from build123d import *

# Parameters (mm, degrees)
SKETCH1_W               = 50
SKETCH1_H               = 91
SKETCH1_W_2             = 37.5
SKETCH1_W_3             = 25
BOSS_EXTRUDE1_DEPTH     = 25
SKETCH1_3_W             = 37.5
SKETCH1_3_H             = 91
BOSS_EXTRUDE2_DEPTH     = 35
BOSS_EXTRUDE3_REACH     = 66.013
SKETCH4_R               = 12.5
SKETCH4_R_2             = 6
SKETCH4_4_R             = 6
CUT_EXTRUDE1_DEPTH      = 65.01307477
SKETCH4_5_R             = 12.5
SKETCH4_5_R_2           = 6
BOSS_EXTRUDE4_DEPTH     = 15
SKETCH5_W               = 91
SKETCH5_H               = 60
BOSS_EXTRUDE5_DEPTH     = 15
CUT_EXTRUDE2_DEPTH      = 1
CUT_EXTRUDE2_DEPTH_BACK = 21
EXTRUDE_THIN1_DEPTH     = 21
BOSS_EXTRUDE6_REACH     = 88.811
SKETCH9_R               = 7.5
CUT_EXTRUDE4_DEPTH      = 5
SKETCH9_6_R             = 12.5
CUT_EXTRUDE5_DEPTH      = 5
SKETCH9_7_R             = 7.5
CUT_EXTRUDE6_DEPTH      = 87.810889132


with BuildPart() as part:
    # Sketch1 → Boss-Extrude1 (new body)
    with BuildSketch(Plane(origin=(0, 0, 0), x_dir=(0, 0, -1), z_dir=(0, 1, 0))):
        with Locations((25, 45.5)):
            Rectangle(SKETCH1_W, SKETCH1_H)
        with Locations((68.75, 45.5)):
            Rectangle(SKETCH1_W_2, SKETCH1_H)
        with Locations((100, 45.5)):
            Rectangle(SKETCH1_W_3, SKETCH1_H)
        with Locations((131.25, 45.5)):
            Rectangle(SKETCH1_W_2, SKETCH1_H)
        with Locations((175, 45.5)):
            Rectangle(SKETCH1_W, SKETCH1_H)
    extrude(amount=-BOSS_EXTRUDE1_DEPTH)

    # Sketch1<3> → Boss-Extrude2 (add)
    with BuildSketch(Plane(origin=(0, 0, 0), x_dir=(0, 0, -1), z_dir=(0, 1, 0))):
        with Locations((68.75, 45.5)):
            Rectangle(SKETCH1_3_W, SKETCH1_3_H)
        with Locations((131.25, 45.5)):
            Rectangle(SKETCH1_3_W, SKETCH1_3_H)
    extrude(amount=-BOSS_EXTRUDE2_DEPTH)

    # Boss-Extrude3: up to this face of the body (flat: up to its plane)
    boss_extrude3_end = Plane(part.part.faces().sort_by_distance((-45.5, 0, -100))[0])
    # Sketch4 → Boss-Extrude3 (add, up to the picked face)
    with BuildSketch(Plane(origin=(0, 0, 0), x_dir=(0.939692621, -0.342020143, 0), z_dir=(0.342020143, 0.939692621, 0)), mode=Mode.PRIVATE) as boss_extrude3_sk1:
        with BuildLine():
            ThreePointArc((-40, 15), (-65, 40), (-40, 65))
            Line((-40, 65), (0, 65))
            Line((0, 65), (0, 15))
            Line((0, 15), (-40, 15))
        make_face()
        with Locations((-40, 40)):
            Circle(SKETCH4_R, mode=Mode.SUBTRACT)
    boss_extrude3_tool1 = split(extrude(boss_extrude3_sk1.sketch, amount=-BOSS_EXTRUDE3_REACH, mode=Mode.PRIVATE), bisect_by=boss_extrude3_end, keep=Keep.BOTH, mode=Mode.PRIVATE)
    add(boss_extrude3_tool1.solids().sort_by_distance((-60.309415, 21.950832, -40))[0])
    # Sketch4 → Boss-Extrude3 (add, up to the picked face)
    with BuildSketch(Plane(origin=(0, 0, 0), x_dir=(0.939692621, -0.342020143, 0), z_dir=(0.342020143, 0.939692621, 0)), mode=Mode.PRIVATE) as boss_extrude3_sk2:
        with Locations((-40, 40)):
            Circle(SKETCH4_R)
        with Locations((-40, 40)):
            Circle(SKETCH4_R_2, mode=Mode.SUBTRACT)
    boss_extrude3_tool2 = split(extrude(boss_extrude3_sk2.sketch, amount=-BOSS_EXTRUDE3_REACH, mode=Mode.PRIVATE), bisect_by=boss_extrude3_end, keep=Keep.BOTH, mode=Mode.PRIVATE)
    add(boss_extrude3_tool2.solids().sort_by_distance((-49.001631, 17.835135, -40))[0])

    # Sketch4<4> → Cut-Extrude1 (cut, through all)
    with BuildSketch(Plane(origin=(0, 0, 0), x_dir=(0.939692621, -0.342020143, 0), z_dir=(0.342020143, 0.939692621, 0))):
        with Locations((-40, 40)):
            Circle(SKETCH4_4_R)
    extrude(amount=-CUT_EXTRUDE1_DEPTH, mode=Mode.SUBTRACT)

    # Sketch4<5> → Boss-Extrude4 (add)
    with BuildSketch(Plane(origin=(0, 0, 0), x_dir=(0.939692621, -0.342020143, 0), z_dir=(0.342020143, 0.939692621, 0))):
        with Locations((-40, 40)):
            Circle(SKETCH4_5_R)
        with Locations((-40, 40)):
            Circle(SKETCH4_5_R_2, mode=Mode.SUBTRACT)
    extrude(amount=BOSS_EXTRUDE4_DEPTH)

    # Sketch5 → Boss-Extrude5 (add)
    with BuildSketch(Plane(origin=(0, 0, 0), x_dir=(1, 0, 0), z_dir=(0, 1, 0))):
        with Locations((-45.5, 170)):
            Rectangle(SKETCH5_W, SKETCH5_H)
    extrude(amount=BOSS_EXTRUDE5_DEPTH)

    # Sketch6 → Cut-Extrude2 (cut, two sides)
    with BuildSketch(Plane(origin=(0, 0, 0), x_dir=(0, 0, -1), z_dir=(1, 0, 0))) as cut_extrude2_sk:
        with BuildLine():
            ThreePointArc((78.205505282, 0), (100, -5), (121.794494718, 0))
            Line((121.794494718, 0), (78.205505282, 0))
        make_face()
    extrude(amount=CUT_EXTRUDE2_DEPTH, mode=Mode.SUBTRACT)
    extrude(cut_extrude2_sk.sketch, amount=-CUT_EXTRUDE2_DEPTH_BACK, mode=Mode.SUBTRACT)

    # Sketch6<2> → Extrude-Thin1 (add)
    with BuildSketch(Plane(origin=(0, 0, 0), x_dir=(0, 0, -1), z_dir=(1, 0, 0))):
        with BuildLine():
            ThreePointArc((78.205505282, 0), (111.794494718, -3.588989435), (140, 15))
            Line((140, 15), (148, 9))
            ThreePointArc((148, 9), (114.153393661, -13.306787322), (73.846606339, -9))
            Line((73.846606339, -9), (78.205505282, 0))
        make_face()
    extrude(amount=-EXTRUDE_THIN1_DEPTH)

    # Sketch9 → Boss-Extrude6 (add, up to next)
    with BuildSketch(Plane(origin=(0, -37.672105065, -21.75), x_dir=(1, 0, 0), z_dir=(0, 0.866025404, 0.5)), mode=Mode.PRIVATE) as boss_extrude6_sk1:
        with BuildLine():
            Line((-21, 75.344210129), (-21, 125.344210129))
            ThreePointArc((-21, 125.344210129), (-56, 160.344210129), (-91, 125.344210129))
            Line((-91, 125.344210129), (-91, 75.344210129))
            Line((-91, 75.344210129), (-21, 75.344210129))
        make_face()
        with Locations((-56, 125.344210129)):
            Circle(SKETCH9_R, mode=Mode.SUBTRACT)
    boss_extrude6_tool1 = extrude(boss_extrude6_sk1.sketch, amount=-BOSS_EXTRUDE6_REACH, mode=Mode.PRIVATE) - part.part
    add(boss_extrude6_tool1.solids().sort_by_distance((-56, 19.386227, -120.577931))[0])

    # Sketch9<5> → Cut-Extrude4 (cut)
    with BuildSketch(Plane(origin=(0, -37.672105065, -21.75), x_dir=(1, 0, 0), z_dir=(0, 0.866025404, 0.5))):
        with BuildLine():
            Line((-44.543560763, 120.344210129), (-21, 120.344210129))
            Line((-21, 120.344210129), (-21, 125.344210129))
            ThreePointArc((-21, 125.344210129), (-21.08986132, 127.850645317), (-21.358983849, 130.344210129))
            Line((-21.358983849, 130.344210129), (-44.543560763, 130.344210129))
            ThreePointArc((-44.543560763, 130.344210129), (-43.5, 125.344210129), (-44.543560763, 120.344210129))
        make_face()
        with BuildLine():
            Line((-61, 75.344210129), (-51, 75.344210129))
            Line((-51, 75.344210129), (-51, 113.887770892))
            ThreePointArc((-51, 113.887770892), (-56, 112.844210129), (-61, 113.887770892))
            Line((-61, 113.887770892), (-61, 75.344210129))
        make_face()
        with BuildLine():
            Line((-51, 136.800649367), (-51, 159.985226281))
            ThreePointArc((-51, 159.985226281), (-56, 160.344210129), (-61, 159.985226281))
            Line((-61, 159.985226281), (-61, 136.800649367))
            ThreePointArc((-61, 136.800649367), (-56, 137.844210129), (-51, 136.800649367))
        make_face()
        with BuildLine():
            Line((-91, 125.344210129), (-91, 120.344210129))
            Line((-91, 120.344210129), (-67.456439237, 120.344210129))
            ThreePointArc((-67.456439237, 120.344210129), (-68.5, 125.344210129), (-67.456439237, 130.344210129))
            Line((-67.456439237, 130.344210129), (-90.641016151, 130.344210129))
            ThreePointArc((-90.641016151, 130.344210129), (-90.91013868, 127.850645317), (-91, 125.344210129))
        make_face()
    extrude(amount=-CUT_EXTRUDE4_DEPTH, mode=Mode.SUBTRACT)

    # Sketch9<6> → Cut-Extrude5 (cut)
    with BuildSketch(Plane(origin=(0, -37.672105065, -21.75), x_dir=(1, 0, 0), z_dir=(0, 0.866025404, 0.5))):
        with Locations((-56, 125.344210129)):
            Circle(SKETCH9_6_R)
    extrude(amount=-CUT_EXTRUDE5_DEPTH, mode=Mode.SUBTRACT)

    # Sketch9<7> → Cut-Extrude6 (cut, through all)
    with BuildSketch(Plane(origin=(0, -37.672105065, -21.75), x_dir=(1, 0, 0), z_dir=(0, 0.866025404, 0.5))):
        with Locations((-56, 125.344210129)):
            Circle(SKETCH9_7_R)
    extrude(amount=-CUT_EXTRUDE6_DEPTH, mode=Mode.SUBTRACT)


solid = part.part
Geometry check sheet. Reference: the model listing, model coordinates, mm. A direction names the side the tool comes from. Coordinates: 2 decimals unless noted, no trailing zeros. Loops run counter-clockwise (first coordinate to the right, second up) from the corner with the lowest first, then second, coordinate; pieces in that order, holes last. Notation, with made-up numbers: (67.25, -25.75) - (123.25, -25.75) arc R19 cw to (123.25, -12.75) - close; hole circle Ø10 at (-8.5, 82). An arc over 180 degrees is marked (long way). Use one line per item in the form item = value. Start each with the question number.
Item 1: Section check D-D, the plane y = -16.5. Give the number of separate pieces and of enclosed holes in the cut face, and give its area (3 significant figures).
Item 2: Section check B-B, the plane z = -93. Enter the section's corners in (x, y), and give its area (3 significant figures).
Item 3: Mould release check, pull along Z, two halves, no side actions. Record for faces 1 (the face through (-64.79, 27.31, -139.23)), 2 (the face through (-32.94, 20.37, -127.2)), 3 (the face through (-45, -30, -150)): +Z half, -Z half, draft (parallel to the pull), parting line (faces both ways), or undercut.
Item 4: Thickness scan on probe 1 along Z at (x, y) = (-51.5, -14.5); probe 2 along Z at (x, y) = (-61.5, -26.5); probe 3 along Z at (x, y) = (-25.5, 22). Record the ranges inside material, lowest first.
Item 5: Section check C-C, the plane z = -115. Enter the section's corners in (x, y).
Item 6: Gauge pin test, flat ends, axial feed: pin 1 (1 mm diameter, centred on y = 10.5, z = -61.5, fed in from -X); pin 2 (8 mm diameter, centred on y = 9.5, z = -115.5, fed in from +X); pin 3 (4 mm diameter, centred on x = -19.5, z = -169.5, fed in from +Y). Record the tip position at first contact, or that the pin passes through.
Item 7: Section check A-A, the plane y = -28. Enter the section's corners in (x, z).
Item 8: Tool access check on faces 4 (the face through (-61, 34, -152)), 5 (the face through (-45, -30, -87.5)), 6 (the face through (-21, 6, -115)), 7 (the face through (-61, 8, -105)), 8 (the face through (-66, 0, -53)). Record the directions out of +Z, -Z, +X, -X, +Y, -Y that give a thin tool (end or side, any length) a straight path to the whole face; none if there is none.
Computed:
q1.separate_pieces = 1
q1.enclosed_holes = 2
q1.area = 17,900 mm2
q2.outline = (-91, -25) - (0, -25) - (0, -4.51) - (-21, -4.51) - (-21, 3.46) - (-51, 3.46) - (-51, -2.31) - (-61, -2.31) - (-61, 3.46) - (-91, 3.46) - close
q2.area = 2,370 mm2
q3.face_1 = +Z half
q3.face_2 = undercut
q3.face_3 = -Z half
q4.probe_1 = -200 to -160.03, -146.18 to -44.92, -35.08 to 0
q4.probe_2 = -150 to -112.5, -87.5 to -50
q4.probe_3 = -151.86 to -135.11, -126.26 to -125.11, -49.15 to -30.85
q5.outline = (-91, -35) - (0, -35) - (0, -2.7) - (-21, -2.7) - (-21, 16.17) - (-51, 16.17) - (-51, 10.39) - (-61, 10.39) - (-61, 16.17) - (-91, 16.17) - close
q6.pin_1 = -53.2
q6.pin_2 = -21
q6.pin_3 = 15
q7.outline = (-91, -150) - (0, -150) - (0, -112.5) - (-91, -112.5) - close; (-91, -87.5) - (0, -87.5) - (0, -50) - (-91, -50) - close
q8.face_4 = +Z, +Y
q8.face_5 = +X, -X, -Y
q8.face_6 = +X, +Y
q8.face_7 = +Y
q8.face_8 = -X, +Y
